Can you work these out from the model? Positions are in its coordinate system, mm. Coordinates: 2 decimals unless noted, no trailing zeros. Loops run counter-clockwise (first coordinate to the right, second up) from the corner with the lowest first, then second, coordinate; pieces in that order, holes last.
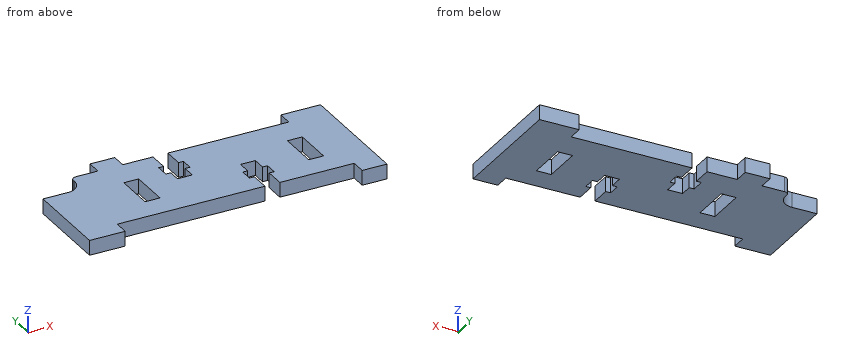
```python
from build123d import *

# Parameters (mm, degrees)
ESQUISSE1_W               = 3
ESQUISSE1_H               = 8
T_LE_DE_BASE_PLI_E1_DEPTH = 3
CONG_1_R                  = 1


# Sheet-metal steps are written as plain solids
with BuildPart() as part:
    # Esquisse1 → Tôle de base pliée1 (new body)
    with BuildSketch(Plane.XY):
        with BuildLine():
            Line((60, 25), (60, 0))
            Line((60, 0), (55, 0))
            Line((55, 0), (55, 3))
            Line((55, 3), (40, 3))
            Line((40, 3), (40, 7))
            Line((40, 7), (41, 7))
            Line((41, 7), (41, 9.5))
            Line((41, 9.5), (40, 9.5))
            Line((40, 9.5), (40, 12.2))
            Line((40, 12.2), (37, 12.2))
            Line((37, 12.2), (37, 9.5))
            Line((37, 9.5), (36, 9.5))
            Line((36, 9.5), (36, 7))
            Line((36, 7), (37, 7))
            Line((37, 7), (37, 3))
            Line((37, 3), (7.2, 3))
            Line((7.2, 3), (7.2, 0))
            Line((7.2, 0), (0, 0))
            Line((0, 0), (0, 17.5))
            Line((0, 17.5), (5, 17.5))
            ThreePointArc((5, 17.5), (7.121320344, 18.378679656), (8, 20.5))
            Line((8, 20.5), (8, 22))
            Line((8, 22), (13.5, 22))
            Line((13.5, 22), (13.5, 25))
            Line((13.5, 25), (18.5, 25))
            Line((18.5, 25), (18.5, 22))
            Line((18.5, 22), (24.6, 22))
            Line((24.6, 22), (24.6, 18))
            Line((24.6, 18), (23.6, 18))
            Line((23.6, 18), (23.6, 15.3))
            Line((23.6, 15.3), (24.6, 15.3))
            Line((24.6, 15.3), (24.6, 12.8))
            Line((24.6, 12.8), (27.6, 12.8))
            Line((27.6, 12.8), (27.6, 15.5))
            Line((27.6, 15.5), (28.6, 15.5))
            Line((28.6, 15.5), (28.6, 18))
            Line((28.6, 18), (27.6, 18))
            Line((27.6, 18), (27.6, 22))
            Line((27.6, 22), (52, 22))
            Line((52, 22), (52, 25))
            Line((52, 25), (60, 25))
        make_face()
        with Locations((17, 12)):
            Rectangle(ESQUISSE1_W, ESQUISSE1_H, mode=Mode.SUBTRACT)
        with Locations((50, 12)):
            Rectangle(ESQUISSE1_W, ESQUISSE1_H, mode=Mode.SUBTRACT)
    extrude(amount=-T_LE_DE_BASE_PLI_E1_DEPTH)

    # Congé1
    cong_1_edges = [part.edges().sort_by_distance(p)[0] for p in [
        (8, 22, -1.5),
    ]]
    fillet(cong_1_edges, radius=CONG_1_R)


solid = part.part
```
Item 1: Suppose I cut it at B-B, the plane y = 10.75. Please give me the cut outline in (x, z), plus the area to 3 significant figures.
Results are:
outline: (0, -3) - (15.5, -3) - (15.5, 0) - (0, 0) - close; (18.5, -3) - (37, -3) - (37, 0) - (18.5, 0) - close; (40, -3) - (48.5, -3) - (48.5, 0) - (40, 0) - close; (51.5, -3) - (60, -3) - (60, 0) - (51.5, 0) - close
area: 153 mm2
Item 2: Suppose I cut it at D-D, the plane x = 26.5. Please give me the cut outline in (y, z).
Results are:
outline: (3, -3) - (12.8, -3) - (12.8, 0) - (3, 0) - close
Item 3: I need wall thicknesses on line 1 along X through (y, z) = (12, -2.3); line 2 along X through (y, z) = (14.5, -0.2); line 3 along Y through (x, z) = (17, -0.8). Which ranges of each line are inside material? Lowest first, please.
Results are:
line 1: x = 0 to 15.5, 18.5 to 37, 40 to 48.5, 51.5 to 60
line 2: x = 0 to 15.5, 18.5 to 24.6, 27.6 to 48.5, 51.5 to 60
line 3: y = 3 to 8, 16 to 25
Item 4: Suppose I cut it at C-C, the plane z = -1.75. Count the separate pieces of the cut face and the enclosed holes in it, plus the area to 3 significant figures.
Results are:
separate pieces: 1
enclosed holes: 2
area: 1,070 mm2
Item 5: I'm going to push flat-ended pins straight in: P1, Ø0.5, axis at x = 40.5, z = -1, coming from the +Y side; P2, Ø0.9, axis at x = 17, z = -1.5, coming from the -Y side; P3, Ø0.9, axis at y = 24, z = -1, coming from the -X side. Where does each tip first touch, or does it pass through?
Results are:
P1: stops at y = 22
P2: stops at y = 3
P3: stops at x = 13.5
Item 6: Suppose I cut it at A-A, the plane y = 23. Please give me the cut outline in (x, z).
Results are:
outline: (13.5, -3) - (18.5, -3) - (18.5, 0) - (13.5, 0) - close; (52, -3) - (60, -3) - (60, 0) - (52, 0) - close
